from build123d import *

# Parameters (mm, degrees)
SKETCH1_W = 7
SKETCH1_H = 7
FILLET1_R = 1


with BuildPart() as part:
    # Sketch1 → Revolve1 (revolve)
    with BuildSketch(Plane.XY):
        with Locations((0, 7.5)):
            Rectangle(SKETCH1_W, SKETCH1_H)
    revolve(axis=Axis((0, 0, 0), (1, 0, 0)))

    # Fillet1
    fillet1_edges = [part.edges().sort_by_distance(p)[0] for p in [
        (-3.5, -4, 0),
        (3.5, -4, 0),
        (3.5, -11, 0),
        (-3.5, -11, 0),
    ]]
    fillet(fillet1_edges, radius=FILLET1_R)


solid = part.part
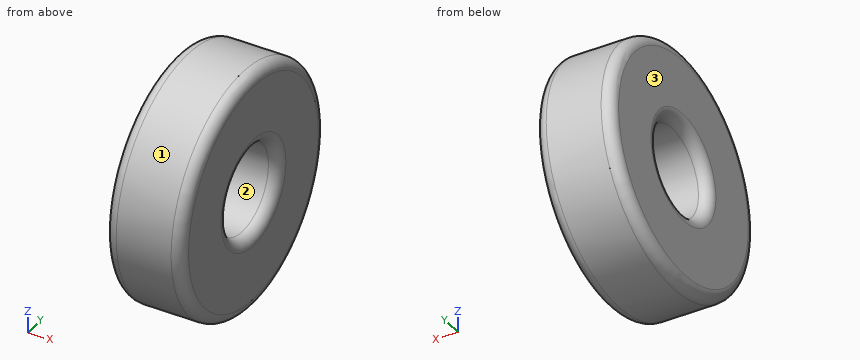
Model file for the job. Use its own axes, mm. Face numbers are marked on the shaded views. Coordinates: 2 decimals unless noted, no trailing zeros. Loops run counter-clockwise (first coordinate to the right, second up) from the corner with the lowest first, then second, coordinate; pieces in that order, holes last. Notation, with made-up numbers: (-30, 85.5) -> (-14, 85.5) arc R16 ccw to (-14, 96.5) -> close; hole circle Ø9 at (-7.5, 84). An arc over 180 degrees is marked (long way). Use one line per item in the form item = value. Start each with the question number.
(1) Probe probe 1 along Z at (x, y) = (1.25, 0); probe 2 along Z at (x, y) = (-1.25, -3.25); probe 3 along Y at (x, z) = (-2, -2.25). List the from-to ranges inside material, lowest first. Write a range as from..to.
(2) Pull direction Y, two halves, no side cores. Call the marked faces 1, 2 and 3: pulls with the +Y half, pulls with the -Y half, needs draft (parallel to the pull), parting line crosses it, or undercut.
(3) Cut at A-A on z = 0. Give the cut face in (x, y), and give its area (3 significant figures).
(4) Cut at C-C on x = 0.5. Give the cut face in (y, z), and give its area (3 significant figures).
(5) Flat gauge pins, fed straight in: pin 1 (1 mm diameter, centred on x = 1, y = -8, fed in from -Z); pin 2 (2 mm diameter, centred on x = 2, y = 9, fed in from -Z); pin 3 (1.5 mm diameter, centred on x = 1.5, z = -2.5, fed in from -Y). Where does each tip first touch, or does it go through?
Values:
q1.probe_1 = -11..-4, 4..11
q1.probe_2 = -10.51..-2.33, 2.33..10.51
q1.probe_3 = -10.77..-3.31, 3.31..10.77
q2.face_1 = parting line crosses it
q2.face_2 = undercut
q2.face_3 = needs draft
q3.outline = (-3.5, -10) arc R1 ccw to (-2.5, -11) -> (2.5, -11) arc R1 ccw to (3.5, -10) -> (3.5, -5) arc R1 ccw to (2.5, -4) -> (-2.5, -4) arc R1 ccw to (-3.5, -5) -> close; (-3.5, 5) arc R1 ccw to (-2.5, 4) -> (2.5, 4) arc R1 ccw to (3.5, 5) -> (3.5, 10) arc R1 ccw to (2.5, 11) -> (-2.5, 11) arc R1 ccw to (-3.5, 10) -> close
q3.area = 96.3 mm2
q4.outline = circle Ø22 at (0, 0); hole circle Ø8 at (0, 0)
q4.area = 330 mm2
q5.pin_1 = -8.05
q5.pin_2 = -7.55
q5.pin_3 = -10.86
